Check sheet for the modelled part. Datum: model origin and axes. Units: mm. Face numbers are marked on the shaded views. Give positions to 0.01 mm unless a question says otherwise; leave off trailing zeros. Write each loop counter-clockwise with the first axis right and the second up, starting at its lowest first coordinate (ties: lowest second). Pieces come first, ordered by that corner, then holes. Notation, with made-up numbers: M 6.25,70.25 L 57.25,70.25 A12 ccw 57.25,81.25 Z; hole C -8.5,-8 d9. An arc over 180 degrees is marked long. Use CSV: the item, a comma, the result in double quotes. Start each with the question number.
1. Depth check by flat-ended pin: P1, Ø6, axis at x = -4.5, y = 97.5, coming from the -Z side; P2, Ø1.5, axis at y = 156, z = 4.5, coming from the +X side; P3, Ø3, axis at y = 87.5, z = 11.5, coming from the +X side. Enter the tip coordinate at first touch or a pass-through.
2. Cross-section at D-D, the plane y = 151.5. Enter the section's corners in (x, z).
3. Cross-section at C-C, the plane x = -17. Enter the section's corners in (y, z), and give its area (3 significant figures).
4. Cross-section at A-A, the plane z = 0. Enter the section's corners in (x, y), and give its area (3 significant figures).
5. Cross-section at B-B, the plane x = 0. Enter the section's corners in (y, z).
6. Scan lines: line 1 (X direction, y = 79, z = 0); line 2 (X direction, y = 116, z = 11). Record each from-to range of solid material in increasing order.
7. Mould release check, pull along Z, two halves, no side actions. Record for the marked faces 1 and 2: +Z half, -Z half, draft (parallel to the pull), parting line (faces both ways), or undercut.
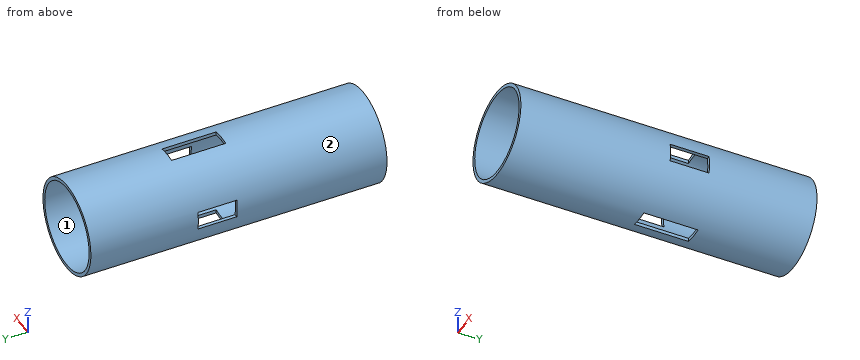
from build123d import *

# Parameters (mm, degrees)
SKETCH1_R               = 27.5
SKETCH1_R_2             = 25.5
BOSS_EXTRUDE1_DEPTH     = 175
CUT_EXTRUDE1_DEPTH      = 180.26935042
CUT_EXTRUDE1_DEPTH_BACK = 180.26935042
SKETCH3_W               = 11
SKETCH3_H               = 23
CUT_EXTRUDE2_DEPTH      = 180.26935042
CUT_EXTRUDE2_DEPTH_BACK = 180.26935042
SKETCH4_W               = 11
SKETCH4_H               = 32


with BuildPart() as part:
    # Sketch1 → Boss-Extrude1 (new body)
    with BuildSketch(Plane(origin=(0, 0, 0), x_dir=(1, 0, 0), z_dir=(0, 1, 0))):
        with Locations(Location((0, 0, 0), (0, 0, 270))):
            Circle(SKETCH1_R)
        with Locations(Location((0, 0, 0), (0, 0, 270))):
            Circle(SKETCH1_R_2, mode=Mode.SUBTRACT)
    extrude(amount=BOSS_EXTRUDE1_DEPTH)

    # Sketch3 → Cut-Extrude1 (cut, two sides: drawn at the far end of the back side and taken through both)
    with BuildSketch(Plane(origin=(0, 0, 0), x_dir=(0, 0, -1), z_dir=(1, 0, 0)).offset(-CUT_EXTRUDE1_DEPTH_BACK)):
        with Locations((0, 100)):
            Rectangle(SKETCH3_W, SKETCH3_H)
    extrude(amount=CUT_EXTRUDE1_DEPTH + CUT_EXTRUDE1_DEPTH_BACK, mode=Mode.SUBTRACT)

    # Sketch4 → Cut-Extrude2 (cut, two sides: drawn at the far end of the back side and taken through both)
    with BuildSketch(Plane.XY.offset(-CUT_EXTRUDE2_DEPTH_BACK)):
        with Locations((0, 100)):
            Rectangle(SKETCH4_W, SKETCH4_H)
    extrude(amount=CUT_EXTRUDE2_DEPTH + CUT_EXTRUDE2_DEPTH_BACK, mode=Mode.SUBTRACT)


solid = part.part
Worked answers:
1,P1,"stops at z = -26.94"
1,P2,"stops at x = 27.24"
1,P3,"stops at x = 25.62"
2,outline,"C 0,0 d55; hole C 0,0 d51"
3,outline,"M 0,-21.62 L 175,-21.62 L 175,-19.01 L 0,-19.01 Z; M 0,19.01 L 175,19.01 L 175,21.62 L 0,21.62 Z"
3,area,"913 mm^2"
4,outline,"M -27.5,0 L -25.5,0 L -25.5,88.5 L -27.5,88.5 Z; M -27.5,111.5 L -25.5,111.5 L -25.5,175 L -27.5,175 Z; M 25.5,0 L 27.5,0 L 27.5,88.5 L 25.5,88.5 Z; M 25.5,111.5 L 27.5,111.5 L 27.5,175 L 25.5,175 Z"
4,area,"608 mm^2"
5,outline,"M 0,-27.5 L 84,-27.5 L 84,-25.5 L 0,-25.5 Z; M 0,25.5 L 84,25.5 L 84,27.5 L 0,27.5 Z; M 116,-27.5 L 175,-27.5 L 175,-25.5 L 116,-25.5 Z; M 116,25.5 L 175,25.5 L 175,27.5 L 116,27.5 Z"
6,line 1,"x = -27.5 to -25.5, 25.5 to 27.5"
6,line 2,"x = -25.2 to -23.01, 23.01 to 25.2"
7,face 1,"undercut"
7,face 2,"parting line"
